Work out the finished part from the listing and answer in its coordinate system (mm). Face numbers are marked on the shaded views. Coordinates: 2 decimals unless noted, no trailing zeros. Loops run counter-clockwise (first coordinate to the right, second up) from the corner with the lowest first, then second, coordinate; pieces in that order, holes last. Notation, with made-up numbers: (-7, 22) -> (48, 22) arc R33 ccw to (48, 54) -> close; hole circle Ø6 at (37.25, 57.25). An arc over 180 degrees is marked (long way). Use a Markdown table: item, result.
from build123d import *

# Parameters (mm, degrees)
BOSS_EXTRUDE1_DEPTH = 50.8
BOSS_EXTRUDE2_DEPTH = 11.43


with BuildPart() as part:
    # Sketch1 → Boss-Extrude1 (new body)
    with BuildSketch(Plane.XY):
        Polygon((-2.037826091, 0), (2.037826091, 0), (4.901371199, -0.364452471), (9.560729749, -0.957463816), (23.681538514, -2.754663947), (32.64962373, -4.768284593), (34.544, -5.892440119), (32.599653531, -9.168965231), (31.225129901, -8.353299221), (23.022216919, -6.511484102), (9.079699287, -4.736975649), (4.420340738, -4.143964304), (1.796344675, -3.81), (-1.796344675, -3.81), (-4.420340738, -4.143964304), (-9.079699287, -4.736975649), (-23.022216919, -6.511484102), (-31.225129901, -8.353299221), (-32.599653531, -9.168965231), (-34.544, -5.892440119), (-32.64962373, -4.768284593), (-23.681538514, -2.754663947), (-9.560729749, -0.957463816), (-4.901371199, -0.364452471), align=None)
    extrude(amount=BOSS_EXTRUDE1_DEPTH)

    # Sketch2 → Boss-Extrude2 (add)
    with BuildSketch(Plane(origin=(0, 0, 0), x_dir=(-1, 0, 0), z_dir=(0, 0, -1))):
        Polygon((23.022216919, -6.511484102), (1.796344675, -3.81), (-1.796344675, -3.81), (-23.022216919, -6.511484102), (-23.681538514, -2.754663947), (-2.037826091, 0), (2.037826091, 0), (23.681538514, -2.754663947), align=None)
    extrude(amount=BOSS_EXTRUDE2_DEPTH)


solid = part.part
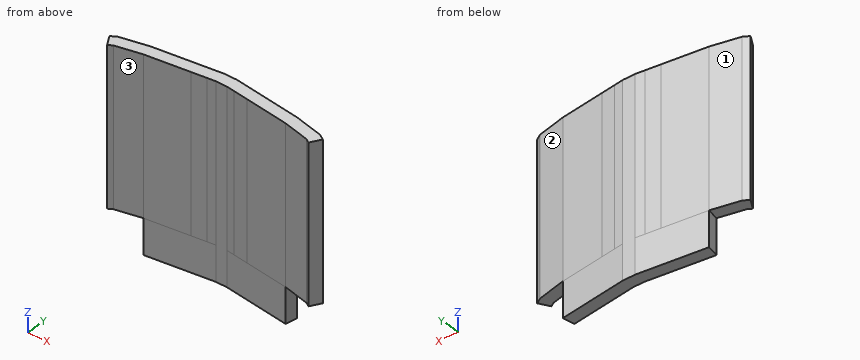
Q1. Section A-A on z = 18.5 is taken. Determine the outline of the cut face in (x, y).
Solved:
| item | result |
|---|---|
| outline | (-34.54, -5.89) -> (-32.6, -9.17) -> (-31.23, -8.35) -> (-23.02, -6.51) -> (-1.8, -3.81) -> (1.8, -3.81) -> (23.02, -6.51) -> (31.23, -8.35) -> (32.6, -9.17) -> (34.54, -5.89) -> (32.65, -4.77) -> (23.68, -2.75) -> (2.04, 0) -> (-2.04, 0) -> (-23.68, -2.75) -> (-32.65, -4.77) -> close |
Q2. Consider line 1 (Y direction, x = -31, z = 46); line 2 (Y direction, x = 4.5, z = -4); line 3 (Z direction, x = 31.5, y = -7.5). Determine where each line is inside the solid, lowest interval first. Write a range as [from, to].
Solved:
| item | result |
|---|---|
| line 1 | [-8.3, -4.4] |
| line 2 | [-4.15, -0.31] |
| line 3 | [0, 50.8] |
Q3. Determine the mould class of the marked faces 1, 2 and 3 for opening direction X: pulls with the +X half, pulls with the -X half, needs draft (parallel to the pull), parting line crosses it, or undercut.
Solved:
| item | result |
|---|---|
| face 1 | pulls with the -X half |
| face 2 | pulls with the +X half |
| face 3 | undercut |
Q4. Section C-C on x = -28 is taken. Determine the outline of the cut face in (y, z).
Solved:
| item | result |
|---|---|
| outline | (-7.63, 0) -> (-3.72, 0) -> (-3.72, 50.8) -> (-7.63, 50.8) -> close |
Q5. Given pin 1 Ø5 at (y, z) = (-7.5, 26) entering from +X; pin 2 Ø2 at (y, z) = (-4, 10.5) entering from -X; pin 3 Ø1.9 at (x, y) = (-30, -6) entering from -Z, each flat-ended and moving along its own axis, determine where each tip first touches the part or whether it passes through.
Solved:
| item | result |
|---|---|
| pin 1 | x = 34.54 |
| pin 2 | x = -33.04 |
| pin 3 | z = 0 |
Q6. Section B-B on x = 6.5 is taken. Determine the outline of the cut face in (y, z), and give its area (3 significant figures).
Solved:
| item | result |
|---|---|
| outline | (-4.41, -11.43) -> (-0.57, -11.43) -> (-0.57, 50.8) -> (-4.41, 50.8) -> close |
| area | 239 mm² |
